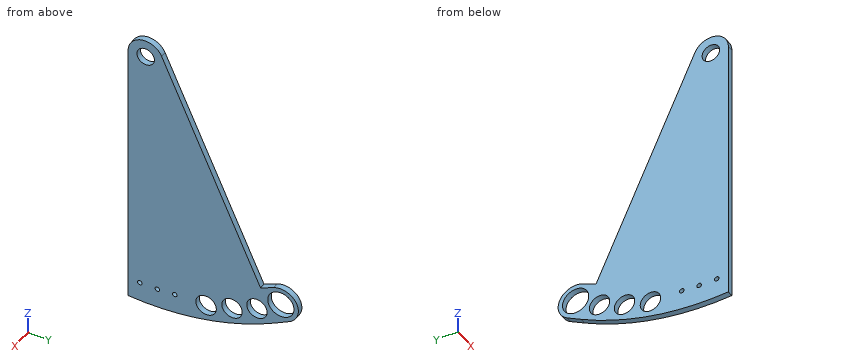
Autodesk Inventor part; units mm, degrees
ref_plane "YZ Plane" through (0, 0, 0) normal (1, 0, 0) x (0, 1, 0)
ref_plane "XZ Plane" through (0, 0, 0) normal (0, 1, 0) x (-1, 0, 0)
ref_plane "XY Plane" through (0, 0, 0) normal (0, 0, 1) x (1, 0, 0)
sketch "Sketch1" plane through (0, 0, 0) normal (1, 0, 0) x (0, 1, 0)
  circle A0 centre (0, 0) radius 9.525
  arc A1 (-25.1608, -265.5105) -> (128.0642, -233.9411) centre (0, 0) ccw construction
  arc A2 (17.3208, 7.9305) -> (-19.05, 0) centre (0, 0) ccw
  line L0 (-19.05, 0) -> (-19.05, -297.8414)
  circle A3 centre (121.0878, -254.0152) radius 14.7 construction
  circle A4 centre (93.9242, -265.2625) radius 14.7 construction
  circle A5 centre (65.7355, -273.6143) radius 14.7 construction
  circle A6 centre (121.0878, -254.0152) radius 11.1125
  circle A7 centre (93.9242, -265.2625) radius 11.1125
  circle A8 centre (65.7355, -273.6143) radius 11.1125
  circle A9 centre (121.0878, -254.0152) radius 12.7 construction
  circle A10 centre (93.9242, -265.2625) radius 12.7 construction
  circle A11 centre (65.7355, -273.6143) radius 12.7 construction
  line L1 (17.3208, 7.9305) -> (125.0203, -227.293)
  arc A12 (-19.05, -276.2038) -> (132.3042, -243.2017) centre (0, 0) ccw construction
  arc A13 (-19.05, -297.8414) -> (141.312, -262.8751) centre (0, 0) ccw
  circle A14 centre (31.6741, -275.0422) radius 2.4892
  circle A15 centre (12.6854, -276.5692) radius 2.4892
  circle A16 centre (-6.3634, -276.7869) radius 2.4892
  arc A17 (-19.05, -286.3871) -> (136.5435, -252.4606) centre (0, 0) ccw construction
  line L2 (0, 0) -> (8.0964, -266.5771) construction
  line L3 (8.4048, -276.7324) -> (8.7133, -286.8877) construction
  line L4 (8.4048, -276.7324) -> (8.0964, -266.5771) construction
  line L5 (51.0397, -273.9694) -> (31.6741, -275.0422) construction
  line L6 (48.6698, -262.2215) -> (54.4639, -293.4384) construction
  line L7 (48.6698, -262.2215) -> (0, 0) construction
  circle A18 centre (147.1034, -238.1338) radius 14.2875
  arc A19 (156.1233, -254.9131) -> (139.1729, -220.813) centre (147.1034, -238.1338) ccw
  line L8 (139.1729, -220.813) -> (125.0203, -227.293)
  line L9 (128.0642, -233.9411) -> (141.312, -262.8751) construction
  line L10 (125.0203, -227.293) -> (128.0642, -233.9411) construction
  line L11 (156.1233, -254.9131) -> (141.312, -262.8751)
  dimension "d0" = 19.05
  dimension "d1" = 266.7
  dimension "d3" = 22.225
  dimension "d4" = 25.4
  dimension "d5" = 2
  dimension "d8" = 9.525
  dimension "d10" = 31.75
  dimension "d11" = 4.9784
  dimension "d12" = 19.05
  dimension "d13" = 19.05
  dimension "d14" = 12.7
  dimension "d17" = 287.02
  dimension "d19" = 19.05
  dimension "d20" = 28.575
  dimension "d22" = 4.7625
  dimension "d24" = 30.48
extrude "Extrusion1" add sketch "Sketch1" along normal blind 6.35
equation "\"d1\" = BallSize + 0.5 * WheelSize - Compression"
properties part number "Shooter Side"
Verification items for the finished model (mm, model axes). Coordinates: 2 decimals unless noted, no trailing zeros. Order: outer loops, then holes, each group sorted by start corner. A loop starts at its lowest first (then second) coordinate and runs counter-clockwise, first axis right, second up. Notation, with made-up numbers: M -2.5,8 L 54.5,8 A11 cw 54.5,28 Z; hole C 69.5,44.5 d5. An arc over 180 degrees is marked long. One line per item, written item: value. Start each with the question number.
Item 1: Sectioned sample at A-A (y = 0). Enter the section's corners in (x, z) (3 decimals), then the cut area to 3 significant figures.
Item 2: Gauge pin test, flat ends, axial feed: pin 1 (1.5 mm diameter, centred on y = 31, z = -160, fed in from -X); pin 2 (3 mm diameter, centred on y = 31.67, z = -275.04, fed in from -X); pin 3 (1 mm diameter, centred on x = 2.5, z = -23.5, fed in from +Y); pin 4 (1 mm diameter, centred on x = 2, y = 3.5, fed in from +Z). Record the tip position at first contact, or that the pin passes through.
Item 3: Sectioned sample at D-D (z = -37.5). Enter the section's corners in (x, y), then the cut area to 3 significant figures.
Item 4: Sectioned sample at B-B (x = 3.5). Count the separate pieces of the cut face and the enclosed holes in it, then the cut area to 3 significant figures.
Item 5: Scan lines: probe 1 along Y at (x, z) = (3.25, -237.5); probe 2 along Y at (x, z) = (5.25, -237); probe 3 along Z at (x, y) = (3.25, 0) (3 decimals). Record each from-to range of solid material in increasing order.
Item 6: Sectioned sample at C-C (y = 136). Enter the section's corners in (x, z).
Conclusion:
1. outline: M 0,-298.45 L 6.35,-298.45 L 6.35,-9.525 L 0,-9.525 Z; M 0,9.525 L 6.35,9.525 L 6.35,19.05 L 0,19.05 Z
1. area: 1,900 mm^2
2. pin 1: stops at x = 0
2. pin 2: passes through
2. pin 3: stops at y = 31.94
2. pin 4: stops at z = 18.81
3. outline: M 0,-19.05 L 6.35,-19.05 L 6.35,38.12 L 0,38.12 Z
3. area: 363 mm^2
4. separate pieces: 1
4. enclosed holes: 8
4. area: 30,000 mm^2
5. probe 1: y = -19.05 to 132.83, 161.38 to 166.14
5. probe 2: y = -19.05 to 132.86, 161.35 to 166.12
5. probe 3: z = -298.45 to -9.525, 9.525 to 19.05
6. outline: M 0,-265.66 L 6.35,-265.66 L 6.35,-247.13 L 0,-247.13 Z; M 0,-229.14 L 6.35,-229.14 L 6.35,-222.27 L 0,-222.27 Z
